```python
from build123d import *

# Parameters (mm, degrees)
F0_R     = 13.85
F1_DEPTH = 30
F2_SIZE  = 4
F3_R     = 1.5875
F4_DEPTH = 14
F5_SIZE  = 2
F6_R     = 1.5
F7_DEPTH = 5


with BuildPart() as f1:
    # F0 (on Top) → F1 (new body)
    with BuildSketch(Plane.XY):
        Circle(F0_R)
    extrude(amount=F1_DEPTH)

    # F2
    f2_edges = [f1.edges().sort_by_distance(p)[0] for p in [
        (-13.85, 0, 30),
    ]]
    chamfer(f2_edges, length=F2_SIZE)

    # F3 (on face) → F4 (join)
    with BuildSketch(Plane.XY.offset(30)):
        Circle(F3_R)
    extrude(amount=F4_DEPTH)

    # F5
    f5_edges = [f1.edges().sort_by_distance(p)[0] for p in [
        (-13.85, 0, 0),
    ]]
    chamfer(f5_edges, length=F5_SIZE)

    # F6 (on face) → F7 (cut)
    with BuildSketch(Plane(origin=(0, 0, 0), x_dir=(1, 0, 0), z_dir=(0, 0, -1))):
        with Locations((5.58971, -5.723211)):
            Circle(F6_R)
        with Locations((6.512679, 6.916286)):
            Circle(F6_R)
        with Locations((-5.601047, 5.712127)):
            Circle(F6_R)
        with Locations((-6.522529, -6.907005)):
            Circle(F6_R)
    extrude(amount=-F7_DEPTH, mode=Mode.SUBTRACT)


solid = f1.part
```
Part model, mm, in its own coordinate system. A direction names the side the tool comes from. Round coordinates to 2 decimals unless told otherwise and drop trailing zeros. Write each loop counter-clockwise with the first axis right and the second up, starting at its lowest first coordinate (ties: lowest second). Pieces come first, ordered by that corner, then holes.
Item 1: Two-plate mould, pull along Y, no slides. Class faces 1 (the flat face through (0, 0, 44)), 2 (the flat face through (6, 6, 5)), 3 (the conical face through (-2.177, -9.805, 29.806)), 4 (the flat face through (-7, 7, 5)): +Y half, -Y half, draft (parallel to the pull), parting line (faces both ways), or undercut.
Results:
face 1: draft
face 2: undercut
face 3: parting line
face 4: undercut
Item 2: Cut at B-B, the plane z = 3.5. Give the cut face in (x, y), plus the area to 3 significant figures.
Results:
outline: circle Ø27.7 at (0, 0); hole circle Ø3 at (-6.52, 6.91); hole circle Ø3 at (-5.6, -5.71); hole circle Ø3 at (5.59, 5.72); hole circle Ø3 at (6.51, -6.92)
area: 574 mm2
Item 3: Probe L1, parallel to Z at x = -3.5, y = -8.25; L2, parallel to Y at x = 7.75, z = 4.5; L3, parallel to Y at x = -0.5, z = 23.5. List the from-to ranges inside material, lowest first.
Results:
L1: z = 0 to 30
L2: y = -11.48 to -7.76, -6.07 to 11.48
L3: y = -13.84 to 13.84
Item 4: Which spindle directions (+Z, -Z, +X, -X, +Y, -Y) get a long thin tool onto all of the face, cutting with end or side? Do faces 5 (the cylindrical face through (6.3, -8.4, 2.5)), 6 (the cylindrical face through (13.21, 4.16, 13.83)), 7 (the cylindrical face through (-0.34, -1.55, 36.9)). Say none if no direction does.
Results:
face 5: -Z
face 6: +Z, -Z
face 7: +Z
Item 5: Cut at A-A, the plane y = 0. Give the cut face in (x, z), plus the area to 3 significant figures.
Results:
outline: (-13.85, 2) - (-11.85, 0) - (11.85, 0) - (13.85, 2) - (13.85, 26) - (9.85, 30) - (1.59, 30) - (1.59, 44) - (-1.59, 44) - (-1.59, 30) - (-9.85, 30) - (-13.85, 26) - close
area: 855 mm2
Item 6: Cut at D-D, the plane z = 10.5. Give the cut face in (x, y).
Results:
outline: circle Ø27.7 at (0, 0)
Item 7: Drop flat-ended pins along their axis: pin 1 Ø4 at (x, y) = (-5.6, -5.71) entering from +Z; pin 2 Ø6 at (x, z) = (-6, 7) entering from +Y; pin 3 Ø1.5 at (x, y) = (-6.5, 6.5) entering from -Z. Give the stop position or say it passes through.
Results:
pin 1: stops at z = 30
pin 2: stops at y = 13.52
pin 3: stops at z = 5
